```python
from build123d import *

# Parameters (mm, degrees)
F5_W        = 30
F5_H        = 40
F6_DEPTH    = 3
F8_D        = 5.5
F9_D        = 3.5
F1_DEPTH    = 25
F2_R        = 3
F3_T1_DEPTH = 23.839434056
F4_T1_DEPTH = 23.839434056


# Not quite as in the source:
# - a fillet or chamfer that OpenCascade refuses, or shapes differently, is made with other operations: its cross-section is extruded or revolved along the edge and cut away or added


with BuildPart() as f6:
    # F5 (on Top) → F6 (new body)
    with BuildSketch(Plane.XY):
        Rectangle(F5_W, F5_H)
    extrude(amount=F6_DEPTH)

    # F8 (through all)
    with Locations(Plane.XY.offset(3)):
        with Locations((-10, 10), (-10, -10)):
            Hole(F8_D / 2)

    # F9 (through all)
    with Locations(Plane.XY.offset(3)):
        with Locations((11, 9.5), (11, -9.5)):
            Hole(F9_D / 2)

    # F0 (on face) → F1 (cut)
    with BuildSketch(Plane.XY.offset(3)):
        with BuildLine():
            Line((-8, -20), (8, -20))
            ThreePointArc((8, -20), (0, -12), (-8, -20))
        make_face()
        with BuildLine():
            ThreePointArc((-8, 20), (0, 12), (8, 20))
            Line((8, 20), (-8, 20))
        make_face()
    extrude(amount=-F1_DEPTH, mode=Mode.SUBTRACT)

    # F2
    f2_edges = [f6.edges().sort_by_distance(p)[0] for p in [
        (15, -20, 1.5),
        (-15, -20, 1.5),
        (15, 20, 1.5),
        (-15, 20, 1.5),
    ]]
    fillet(f2_edges, radius=F2_R)

    # F3: chamfer of 5 on 2 edges, made by hand

    # F3_s2 → F3_t1 (cut)
    with BuildSketch(Plane.XY.offset(-10.419717028)):
        with BuildLine():
            Line((-12, 20), (-7.3846153846, 16.9230769231))
            ThreePointArc((-7.3846153846, 16.9230769231), (-7.8300507328, 18.3597849159), (-8, 20))
            Line((-8, 20), (-12, 20))
        make_face()
        with BuildLine():
            Line((7.3846153846, 16.9230769231), (12, 20))
            Line((12, 20), (8, 20))
            ThreePointArc((8, 20), (7.8300507328, 18.3597849159), (7.3846153846, 16.9230769231))
        make_face()
    extrude(amount=F3_T1_DEPTH, mode=Mode.SUBTRACT)

    # F4: chamfer of 5 on 2 edges, made by hand

    # F4_s2 → F4_t1 (cut)
    with BuildSketch(Plane.XY.offset(-10.419717028)):
        with BuildLine():
            Line((7.3846153846, -16.9230769231), (12, -20))
            Line((12, -20), (8, -20))
            ThreePointArc((8, -20), (7.8300507328, -18.3597849159), (7.3846153846, -16.9230769231))
        make_face()
        with BuildLine():
            Line((-12, -20), (-7.3846153846, -16.9230769231))
            ThreePointArc((-7.3846153846, -16.9230769231), (-7.8300507328, -18.3597849159), (-8, -20))
            Line((-8, -20), (-12, -20))
        make_face()
    extrude(amount=F4_T1_DEPTH, mode=Mode.SUBTRACT)


solid = f6.part
```
Source: CAD feature listing. Evaluate the final solid. Frame: model axes, mm. A direction names the side the tool comes from. Round coordinates to 2 decimals unless told otherwise and drop trailing zeros. Loops run counter-clockwise (first coordinate to the right, second up) from the corner with the lowest first, then second, coordinate; pieces in that order, holes last. Notation, with made-up numbers: M -11.5,61.25 L 29.5,61.25 A18 cw 29.5,90.25 Z; hole C -23,-9.5 d1. An arc over 180 degrees is marked long. Put each result on its own line as item: value.
(1) Section C-C, the plane z = 2.3. Return loops of the section in (x, y).
Solutions:
outline: M -15,-17 A3 ccw -12,-20 L -7.38,-16.92 A8 cw 7.38,-16.92 L 12,-20 A3 ccw 15,-17 L 15,17 A3 ccw 12,20 L 7.38,16.92 A8 cw -7.38,16.92 L -12,20 A3 ccw -15,17 Z; hole C -10,-10 d5.5; hole C -10,10 d5.5; hole C 11,-9.5 d3.5; hole C 11,9.5 d3.5
(2) Section B-B, the plane y = 9.5. Return loops of the section in (x, z), and give its area (3 significant figures).
Solutions:
outline: M -15,0 L -12.7,0 L -12.7,3 L -15,3 Z; M -7.3,0 L 9.25,0 L 9.25,3 L -7.3,3 Z; M 12.75,0 L 15,0 L 15,3 L 12.75,3 Z
area: 63.3 mm²
(3) Ray query, line 1 (Y direction, x = 11, z = 1.05); line 2 (Y direction, x = -9.25, z = 0.6); line 3 (X direction, y = 11, z = 0.7). Return the intervals inside material, ascending. Write a range as [from, to].
Solutions:
line 1: [-19.33, -11.25], [-7.75, 7.75], [11.25, 19.33]
line 2: [-18.17, -12.65], [-7.35, 7.35], [12.65, 18.17]
line 3: [-15, -12.56], [-7.44, 10.1], [11.9, 15]
(4) Section D-D, the plane y = 14.5. Return loops of the section in (x, z).
Solutions:
outline: M -15,0 L -5.81,0 L -5.81,3 L -15,3 Z; M 5.81,0 L 15,0 L 15,3 L 5.81,3 Z
(5) Access query for faces 1 (the face through (15, 0, 1)), 2 (the face through (-9.72, 18.48, 1.48)), 3 (the face through (-9.72, -18.48, 1.48)). Directions: +Z, -Z, +X, -X, +Y, -Y. A direction counts if a zero-diameter tool reaches every point of the face in a straight line with its end or side. Return the directions, or none.
Solutions:
face 1: +Z, -Z, +X, +Y, -Y
face 2: +Z, -Z, +Y
face 3: +Z, -Z, -Y
(6) Section A-A, the plane x = 10. Return loops of the section in (y, z).
Solutions:
outline: M -18.67,0 L -10.94,0 L -10.94,3 L -18.67,3 Z; M -8.06,0 L 8.06,0 L 8.06,3 L -8.06,3 Z; M 10.94,0 L 18.67,0 L 18.67,3 L 10.94,3 Z
(7) Pull-direction query (X, two-part tool) for faces 4 (the face through (14.1, 19.14, 1.52)), 5 (the face through (9.66, -18.44, 1.48)), 6 (the face through (-11.48, 12.32, 1.48)), 7 (the face through (-14.14, 19.1, 1.52)); classes: released by +X, released by -X, zero draft, split by the parting line, or undercut.
Solutions:
face 4: released by +X
face 5: undercut
face 6: undercut
face 7: released by -X
